The listing builds one solid part. Answer for the finished solid, in the listing's coordinates (mm). Face numbers are marked on the shaded views. Give positions to 0.01 mm unless a question says otherwise; leave off trailing zeros. Order: outer loops, then holes, each group sorted by start corner. A loop starts at its lowest first (then second) coordinate and runs counter-clockwise, first axis right, second up. Notation, with made-up numbers: (-38.5, 61) -> (-34.5, 61) arc R17 ccw to (-34.5, 79) -> close; hole circle Ø9 at (45.25, 33.25). An arc over 180 degrees is marked (long way). Answer as a JSON object with one key per item and string values. Group by question number.
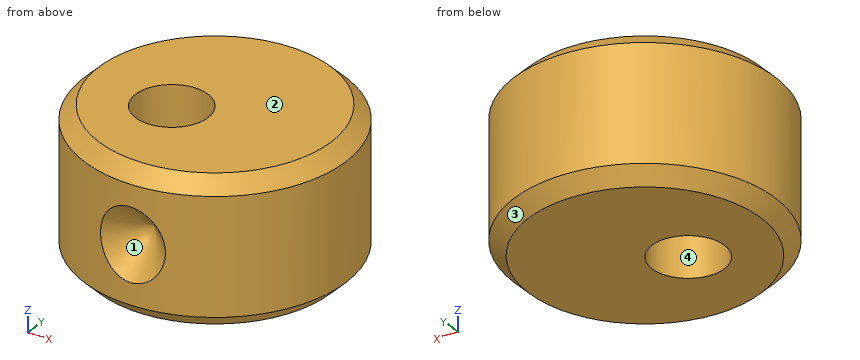
```python
from build123d import *

# Parameters (mm, degrees)
SKETCH_1_R         = 9
EXTRUDE_1_DEPTH    = 5
CHAMFER_1_SIZE     = 1
HOLE_WIZARD_M6_1_D = 5


with BuildPart() as part:
    # 草图1 → 凸台-拉伸1 (new, symmetric)
    with BuildSketch(Plane.XY):
        Circle(SKETCH_1_R)
    extrude(amount=EXTRUDE_1_DEPTH, both=True)

    # 倒角1
    chamfer_1_edges = [part.edges().sort_by_distance(p)[0] for p in [
        (-9, 0, -5),
        (-9, 0, 5),
    ]]
    chamfer(chamfer_1_edges, length=CHAMFER_1_SIZE)

    # M6 螺纹孔1 (through all)
    with Locations(Plane.XY.offset(5)):
        with Locations((-2, -1.5)):
            Hole(HOLE_WIZARD_M6_1_D / 2)

    # 草图5 → 切除-旋转1 (revolve, cut)
    with BuildSketch(Plane(origin=(0, 0, 0), x_dir=(0, 0, -1), z_dir=(1, 0, 0))):
        Polygon((0, -9), (0, -6.5), (2.5, -9), align=None)
    revolve(axis=Axis((0, -9, 0), (0, 1, 0)), mode=Mode.SUBTRACT)


solid = part.part
```
(1) A cutting plane is placed at A-A (y = 0). Determine the outline of the cut face in (x, z).
(2) Find the intervals of material crossed by line 1 along Y through (x, z) = (-4, -2.5); line 2 along X through (y, z) = (-2.75, -1.5); line 3 along Y through (x, z) = (-2, 2), in increasing order. Write a range as [from, to].
(3) Flat-ended cylindrical pins translate along their axes: pin 1 Ø2 at (x, z) = (5.5, 1) entering from -Y; pin 2 Ø4 at (x, y) = (-2, -1.5) entering from +Z; pin 3 Ø5 at (x, z) = (-3, -0.5) entering from +Y; pin 4 Ø3 at (x, y) = (-3.5, -3) entering from +Z. Find the tip coordinate at first contact, or state that the pin passes through.
(4) For a pull along Y with two mould halves and no side action, classify the marked faces 1, 2, 3 and 4 as +Y half, -Y half, draft (parallel to the pull), parting line (faces both ways), or undercut.
Check sheet entries:
{
 "1": {"outline": "(-9, -4) -> (-8, -5) -> (-4, -5) -> (-4, 5) -> (-8, 5) -> (-9, 4) -> close; (0, -5) -> (8, -5) -> (9, -4) -> (9, 4) -> (8, 5) -> (0, 5) -> close"},
 "2": {"line 1": "y = [-8.06, -3], [0, 8.06]", "line 2": "x = [-8.57, -4.17], [0.17, 8.57]", "line 3": "y = [-8.77, -4], [1, 8.77]"},
 "3": {"pin 1": "stops at y = -7.79", "pin 2": "passes through", "pin 3": "stops at y = 8.99", "pin 4": "stops at z = 5"},
 "4": {"face 1": "-Y half", "face 2": "draft", "face 3": "parting line", "face 4": "undercut"}
}
